Source: three-view drawing plus pictorial views. Frame: mm from the lowest corner of the part. Give positions to 0.01 mm unless a question says otherwise; leave off trailing zeros. Order: outer loops, then holes, each group sorted by start corner. A loop starts at its lowest first (then second) coordinate and runs counter-clockwise, first axis right, second up.
1) Draft query along Z for the marked faces 1 and 2. Return one class per face: released by +Z, released by -Z, zero draft, split by the parting line, or undercut.
2) Section A-A, the plane z = 37.5. Return loops of the section in (x, y), plus the area to 3 significant figures.
3) First-contact query: P1, Ø4, axis at x = 20, z = 10, coming from the -Y side; P2, Ø1.5, axis at x = 56, y = 3, coming from the -Z side; P3, Ø6, axis at x = 54.5, y = 4, coming from the -Z side; P4, Ø5, axis at x = 66, y = 21, coming from the -Z side. Flat tips, straight axial feed; report the tip coordinate or a pass-through.
4) Section C-C, the plane x = 64.5. Return loops of the section in (y, z).
5) Section D-D, the plane z = 19. Return loops of the section in (x, y), plus the area to 3 significant figures.
6) Material intervals for line 1 (X direction, y = 6, z = 37.5); line 2 (Z direction, x = 39, y = 22.75); line 3 (Z direction, x = 62.5, y = 23), sorted ascending.
7) Section B-B, the plane y = 7. Return loops of the section in (x, z), plus the area to 3 significant figures.
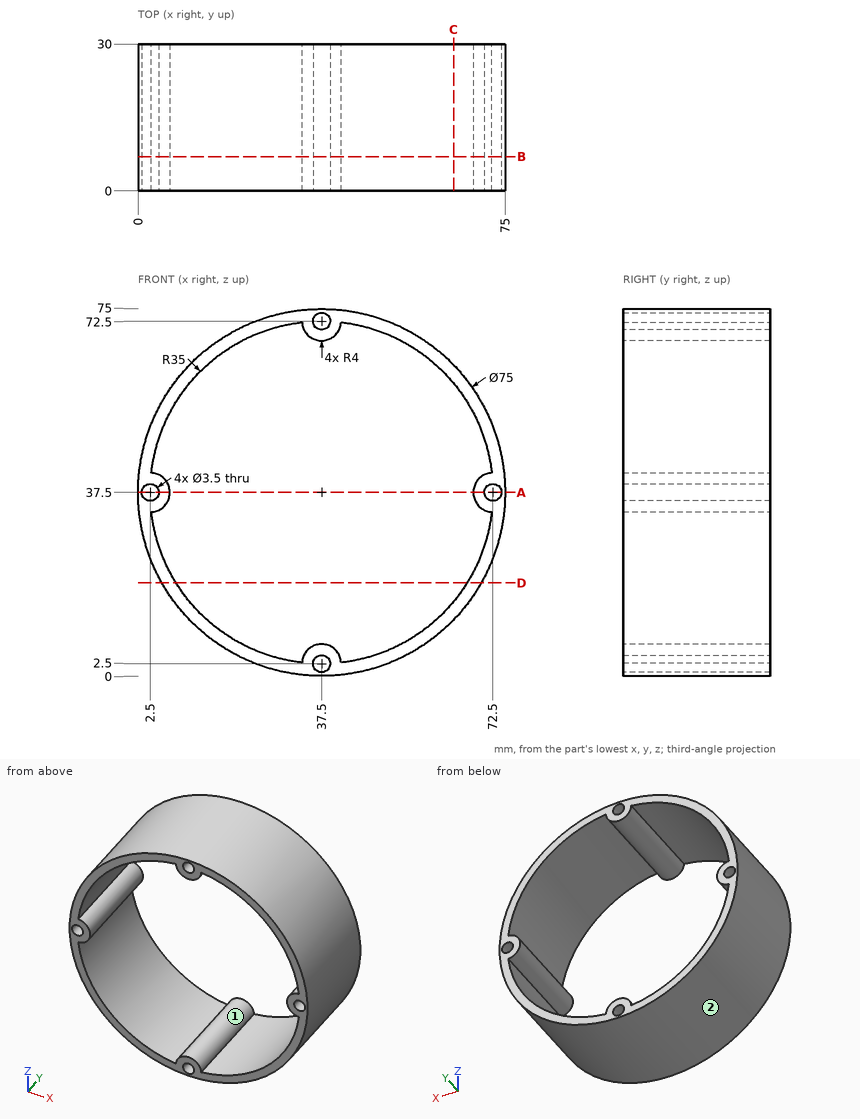
From the geometry:
1. face 1: undercut
1. face 2: split by the parting line
2. outline: (0, 0) - (0.75, 0) - (0.75, 30) - (0, 30) - close; (4.25, 0) - (6.5, 0) - (6.5, 30) - (4.25, 30) - close; (68.5, 0) - (70.75, 0) - (70.75, 30) - (68.5, 30) - close; (74.25, 0) - (75, 0) - (75, 30) - (74.25, 30) - close
2. area: 180 mm2
3. P1: passes through
3. P2: stops at z = 4.47
3. P3: stops at z = 2.71
3. P4: stops at z = 10.48
4. outline: (0, 11.48) - (30, 11.48) - (30, 15.23) - (0, 15.23) - close; (0, 59.77) - (30, 59.77) - (30, 63.52) - (0, 63.52) - close
5. outline: (4.88, 0) - (7.79, 0) - (7.79, 30) - (4.88, 30) - close; (67.21, 0) - (70.12, 0) - (70.12, 30) - (67.21, 30) - close
5. area: 174 mm2
6. line 1: x = 0 to 0.75, 4.25 to 6.5, 68.5 to 70.75, 74.25 to 75
6. line 2: z = 0.03 to 1.6, 3.4 to 6.21, 68.79 to 71.6, 73.4 to 74.97
6. line 3: z = 9.55 to 13.01, 61.99 to 65.45
7. outline: circle Ø75 at (37.5, 37.5); hole circle Ø3.5 at (2.5, 37.5); hole (2.73, 33.51) arc R35 ccw to (33.51, 2.73) arc R4 cw to (41.49, 2.73) arc R35 ccw to (72.27, 33.51) arc R4 cw to (72.27, 41.49) arc R35 ccw to (41.49, 72.27) arc R4 cw to (33.51, 72.27) arc R35 ccw to (2.73, 41.49) arc R4 cw to start; hole circle Ø3.5 at (37.5, 2.5); hole circle Ø3.5 at (37.5, 72.5); hole circle Ø3.5 at (72.5, 37.5)
7. area: 629 mm2
